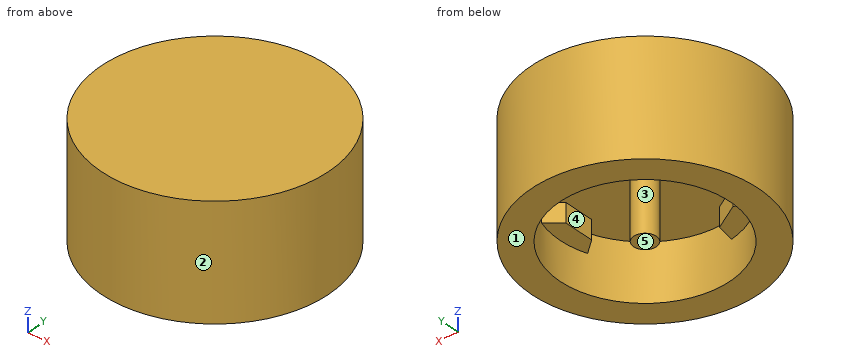
```python
from build123d import *

# Parameters (mm, degrees)
F0_W     = 3.81
F0_H     = 19.05
F3_DEPTH = 6.35


with BuildPart() as f1:
    # F0 (on Front) → F1 (revolve)
    with BuildSketch(Plane.XZ):
        Polygon((0, 19.05), (0, 0), (3.81, 0), (28.575, 0), (28.575, -19.05), (38.1, -19.05), (38.1, 19.05), align=None)
        with Locations((1.905, -9.525)):
            Rectangle(F0_W, F0_H)
    revolve(axis=Axis((0, 0, 9.525), (0, 0, -1)))

    # F2 (on face) → F3 (join)
    with BuildSketch(Plane(origin=(0, 0, 0), x_dir=(1, 0, 0), z_dir=(0, 0, -1))):
        with BuildLine():
            Line((-6.7130909488, 21.7874145991), (-5.5522246622, 28.030401822))
            ThreePointArc((-5.5522246622, 28.030401822), (-14.2875, 24.7466759131), (-21.498927725, 18.823568516))
            Line((-21.498927725, 18.823568516), (-15.5119090512, 16.7074145991))
            Line((-15.5119090512, 16.7074145991), (-11.1125, 19.2474145991))
            Line((-11.1125, 19.2474145991), (-6.7130909488, 21.7874145991))
        make_face()
        with BuildLine():
            Line((22.225, 0), (28.575, 0))
            ThreePointArc((28.575, 0), (28.1914641733, 4.6660446599), (27.0511523872, 9.206833306))
            Line((27.0511523872, 9.206833306), (22.225, 5.08))
            Line((22.225, 5.08), (22.225, 0))
        make_face()
        with BuildLine():
            ThreePointArc((27.0511523872, -9.206833306), (28.1914641733, -4.6660446599), (28.575, 0))
            Line((28.575, 0), (22.225, 0))
            Line((22.225, 0), (22.225, -5.08))
            Line((22.225, -5.08), (27.0511523872, -9.206833306))
        make_face()
        with BuildLine():
            ThreePointArc((-21.498927725, -18.823568516), (-14.2875, -24.7466759131), (-5.5522246622, -28.030401822))
            Line((-5.5522246622, -28.030401822), (-6.7130909488, -21.7874145991))
            Line((-6.7130909488, -21.7874145991), (-11.1125, -19.2474145991))
            Line((-11.1125, -19.2474145991), (-15.5119090512, -16.7074145991))
            Line((-15.5119090512, -16.7074145991), (-21.498927725, -18.823568516))
        make_face()
    extrude(amount=F3_DEPTH)


solid = f1.part
```
The listing builds one solid part. Answer for the finished solid, in the listing's coordinates (mm). Face numbers are marked on the shaded views. A direction names the side the tool comes from. Coordinates: 2 decimals unless noted, no trailing zeros. Write each loop counter-clockwise with the first axis right and the second up, starting at its lowest first coordinate (ties: lowest second). Pieces come first, ordered by that corner, then holes. Notation, with made-up numbers: (22, 12.5) -> (75, 12.5) arc R16 cw to (75, 21.5) -> close; hole circle Ø4 at (41, -6.75). An arc over 180 degrees is marked (long way). Write each question's results on one line, items separated by ' | '. Start each with the question number.
1) Flat-ended cylindrical pins translate along their axes: pin 1 Ø2 at (y, z) = (8, 4.5) entering from -X; pin 2 Ø10 at (x, z) = (-3, 10.5) entering from +Y; pin 3 Ø10 at (y, z) = (-18.5, -7.5) entering from +X. Find the tip coordinate at first contact, or state that the pin passes through.
2) A cutting plane is placed at B-B (x = 0). Determine the outline of the cut face in (y, z) (3 decimals).
3) For a pull along Y with two mould halves and no side action, classify the marked faces 1, 2 and 3 as +Y half, -Y half, draft (parallel to the pull), parting line (faces both ways), or undercut.
4) A cutting plane is placed at A-A (y = 0). Determine the outline of the cut face in (x, z) (3 decimals).
5) A cutting plane is placed at D-D (x = -12). Determine the outline of the cut face in (y, z).
6) Straight lines are drawn through the part: probe 1 along Y at (x, z) = (0, -9) (3 decimals); probe 2 along Z at (x, y) = (6, 0.5). For each, find the intervals that lie inside material, in ascending order.
7) A tool of negligible diameter and unlimited length cuts with its end or side. For the marked faces 4 and 5, from which of +Z, -Z, +X, -X, +Y, -Y can it reach the whole face along a straight path? Write none if from no direction.
8) A cutting plane is placed at C-C (z = 12.5). Determine the outline of the cut face in (x, y).
Values follow:
1) pin 1: x = -37.45 | pin 2: y = 38.1 | pin 3: x = 35.63
2) outline: (-38.1, -19.05) -> (-28.575, -19.05) -> (-28.575, 0) -> (-3.81, 0) -> (-3.81, -19.05) -> (3.81, -19.05) -> (3.81, 0) -> (28.575, 0) -> (28.575, -19.05) -> (38.1, -19.05) -> (38.1, 19.05) -> (-38.1, 19.05) -> close
3) face 1: draft | face 2: parting line | face 3: undercut
4) outline: (-38.1, -19.05) -> (-28.575, -19.05) -> (-28.575, 0) -> (-3.81, 0) -> (-3.81, -19.05) -> (3.81, -19.05) -> (3.81, 0) -> (22.225, 0) -> (22.225, -6.35) -> (28.575, -6.35) -> (28.575, -19.05) -> (38.1, -19.05) -> (38.1, 19.05) -> (-38.1, 19.05) -> close
5) outline: (-36.16, -19.05) -> (-25.93, -19.05) -> (-25.93, -6.35) -> (-18.74, -6.35) -> (-18.74, 0) -> (18.74, 0) -> (18.74, -6.35) -> (25.93, -6.35) -> (25.93, -19.05) -> (36.16, -19.05) -> (36.16, 19.05) -> (-36.16, 19.05) -> close
6) probe 1: -38.1 to -28.575, -3.81 to 3.81, 28.575 to 38.1 | probe 2: 0 to 19.05
7) face 4: -Z | face 5: -Z, +X, -X, +Y, -Y
8) outline: circle Ø76.2 at (0, 0)
